Autodesk Inventor part; units mm, degrees
ref_plane "YZ Plane" through (0, 0, 0) normal (1, 0, 0) x (0, 1, 0)
ref_plane "XZ Plane" through (0, 0, 0) normal (0, 1, 0) x (-1, 0, 0)
ref_plane "XY Plane" through (0, 0, 0) normal (0, 0, 1) x (1, 0, 0)
sketch "Sketch1" plane through (0, 0, 0) normal (1, 0, 0) x (0, 1, 0)
  line L0 (-11.8519, 0.5556) -> (-11.8519, -49.4444)
  line L1 (-11.8519, -49.4444) -> (-7.8519, -49.4444)
  line L2 (-7.8519, -49.4444) -> (-7.8519, 1.5556)
  line L3 (-13.8519, 7.5556) -> (-43.8519, 7.5556)
  line L4 (-43.8519, 7.5556) -> (-43.8519, 3.5556)
  line L5 (-43.8519, 3.5556) -> (-13.8519, 3.5556)
  arc A0 (-7.8519, 1.5556) -> (-13.8519, 7.5556) centre (-13.5586, 1.8488) ccw
  arc A1 (-11.8519, 0.5556) -> (-13.8519, 3.5556) centre (-14.3519, 1.0556) ccw
  point P0 (0, 0)
  dimension "d0" = 4
  dimension "d1" = 4
  dimension "d2" = 50
  dimension "d3" = 57
  dimension "d4" = 30
  dimension "d18" = 30
extrude "Extrusion1" add sketch "Sketch1" along normal blind 30
sketch "Sketch2" plane through (0, -7.8519, 1.5556) normal (0, 1, 0) x (1, 0, 0)
  circle A0 centre (15, 36) radius 3.1
  line L0 (30, 51) -> (30, 0)
  line L1 (0, -6) -> (30, -6)
  point P0 (0, 1.5556)
  dimension "d8" = 6.2
  dimension "d9" = 15
  dimension "d10" = 42
extrude "Extrusion2" cut sketch "Sketch2" against normal blind 30
sketch "Sketch3" plane through (0, -43.8519, 7.5556) normal (0, 0, 1) x (1, 0, 0)
  circle A0 centre (15, 10) radius 3.1
  line L0 (30, 30) -> (30, 0)
  line L1 (0, 0) -> (30, 0)
  point P0 (0, 43.8519)
  dimension "d13" = 6.2
  dimension "d14" = 15
  dimension "d15" = 10
extrude "Extrusion3" cut sketch "Sketch3" against normal blind 30
properties part number "Slider Holding Bracket"
Geometry check sheet. Reference: the model listing, model coordinates, mm. A direction names the side the tool comes from. Round coordinates to 2 decimals unless told otherwise and drop trailing zeros. Loops run counter-clockwise (first coordinate to the right, second up) from the corner with the lowest first, then second, coordinate; pieces in that order, holes last. Notation, with made-up numbers: (-0.5, -39) - (41.5, -39) arc R22 cw to (41.5, -3) - close; hole circle Ø11 at (-30.5, -7). An arc over 180 degrees is marked (long way). Write item = value, one per line. Start each with the question number.
1. Set-up check for faces 4 (the face through (14.79, -12.246, 2.493)), 5 (the face through (15, -29, 3.556)): record each of +Z, -Z, +X, -X, +Y, -Y from which the full face is reachable in a straight line by a thin tool's end or side.
2. Section check C-C on x = 23.75. Enter the section's corners in (y, z), then the cut area to 3 significant figures.
3. Depth check by flat-ended pin: pin 1 (15 mm diameter, centred on x = 22.5, y = -22, fed in from -Z); pin 2 (1.5 mm diameter, centred on x = 4.5, z = -24, fed in from +Y); pin 3 (10 mm diameter, centred on x = 13, y = -33.5, fed in from +Z); pin 4 (5 mm diameter, centred on x = 15, z = -34.44, fed in from +Y) (1 decimal). Enter the tip coordinate at first touch or a pass-through.
4. Mould release check, pull along X, two halves, no side actions. Record for faces 1 (the face through (15, -7.852, -24)), 2 (the face through (0, -11, -12)), 3 (the face through (16.67, -31.24, 5.58)): released by +X, released by -X, zero draft, split by the parting line, or undercut.
5. Section check B-B on y = -36. Enter the section's corners in (x, z).
6. Section check A-A on x = 15. Enter the section's corners in (y, z).
7. Thickness scan on line 1 (Y direction, x = 23.75, z = -41.5); line 2 (Z direction, x = 15, y = -10); line 3 (Z direction, x = 16.5, y = -18). Record the ranges inside material, lowest first.
8. Section check D-D on z = -27. Enter the section's corners in (x, y).
Working result:
q1.face_4 = +X, -X, -Y
q1.face_5 = -Z, +X, -X, -Y
q2.outline = (-43.85, 3.56) - (-13.85, 3.56) arc R2.55 cw to (-11.85, 0.56) - (-11.85, -49.44) - (-7.85, -49.44) - (-7.85, 1.56) arc R5.71 ccw to (-13.85, 7.56) - (-43.85, 7.56) - close
q2.area = 350 mm^2
q3.pin_1 = 3.56
q3.pin_2 = -7.85
q3.pin_3 = 7.56
q3.pin_4 = through
q4.face_1 = zero draft
q4.face_2 = released by -X
q4.face_3 = undercut
q5.outline = (0, 3.56) - (12.76, 3.56) - (12.76, 7.56) - (0, 7.56) - close; (17.24, 3.56) - (30, 3.56) - (30, 7.56) - (17.24, 7.56) - close
q6.outline = (-43.85, 3.56) - (-36.95, 3.56) - (-36.95, 7.56) - (-43.85, 7.56) - close; (-30.75, 3.56) - (-13.85, 3.56) arc R2.55 cw to (-11.85, 0.56) - (-11.85, -31.34) - (-7.85, -31.34) - (-7.85, 1.56) arc R5.71 ccw to (-13.85, 7.56) - (-30.75, 7.56) - close; (-11.85, -49.44) - (-7.85, -49.44) - (-7.85, -37.54) - (-11.85, -37.54) - close
q7.line_1 = -11.85 to -7.85
q7.line_2 = -49.44 to -37.54, -31.34 to 6.32
q7.line_3 = 3.56 to 7.56
q8.outline = (0, -11.85) - (30, -11.85) - (30, -7.85) - (0, -7.85) - close
